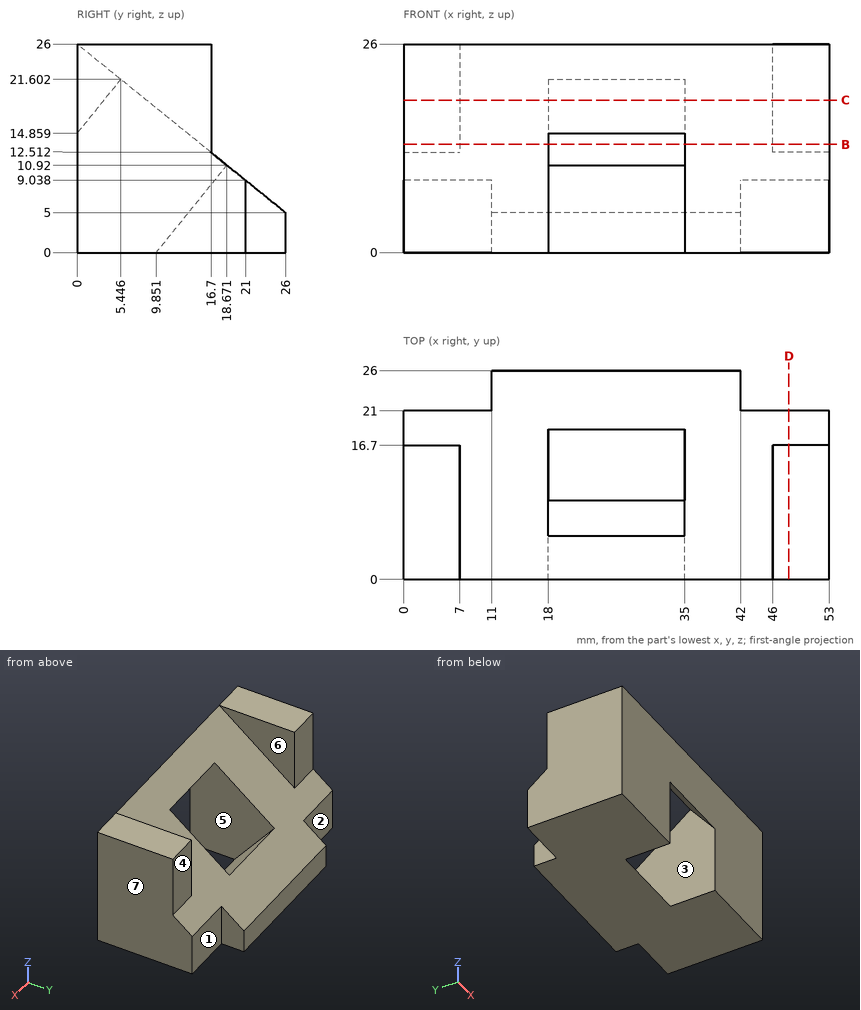
Could you check a few things on this drawing? It's one solid part, dimensions in mm from its lowest x, y, z. A direction names the side the tool comes from. Coordinates: 2 decimals unless noted, no trailing zeros. Order: outer loops, then holes, each group sorted by start corner. A loop starts at its lowest first (then second) coordinate and runs counter-clockwise, first axis right, second up.
1. For the marked faces 1, 2 and 3, which set-ups out of +Z, -Z, +X, -X, +Y, -Y let a thin tool reach every point of the face, with its end or its side?
2. If we section it at D-D (x = 48): Please give me the cut outline in (y, z).
3. If we section it at B-B (z = 13.5): Please give me the cut outline in (x, y), then the cut area to 3 significant figures.
4. I need wall thicknesses on line 1 (X direction, y = 12.25, z = 13.25); line 2 (X direction, y = 16.25, z = 15.75); line 3 (Z direction, x = 35.5, y = 20) (1 decimal). Which ranges of each line are inside material? Lowest first, please.
5. If we section it at C-C (z = 19): Please give me the cut outline in (x, y) (1 decimal).
6. I'm going to push flat-ended pins straight in: pin 1 (5.5 mm diameter, centred on x = 5, z = 17.5, fed in from +Y); pin 2 (1 mm diameter, centred on x = 11.5, z = 6, fed in from +Y); pin 3 (2.5 mm diameter, centred on x = 48.5, z = 5, fed in from +Y). Where does each tip first touch, or does it pass through?
7. Thinking about a two-plate mould opening in X: for the marked faces 4, 5, 6 and 7, which applies, +X half, -X half, draft (parallel to the pull), parting line (faces both ways), or undercut?
Entries:
1. face 1: +Z, -Z, +X, +Y
1. face 2: +Z, -Z, -X, +Y
1. face 3: none
2. outline: (0, 0) - (21, 0) - (21, 9.04) - (16.7, 12.51) - (16.7, 26) - (0, 26) - close
3. outline: (0, 0) - (18, 0) - (18, 15.48) - (7, 15.48) - (7, 16.7) - (0, 16.7) - close; (35, 0) - (53, 0) - (53, 16.7) - (46, 16.7) - (46, 15.48) - (35, 15.48) - close
3. area: 574 mm2
4. line 1: x = 0 to 18, 35 to 53
4. line 2: x = 0 to 7, 46 to 53
4. line 3: z = 0 to 9.8
5. outline: (0, 0) - (53, 0) - (53, 16.7) - (46, 16.7) - (46, 8.7) - (35, 8.7) - (35, 3.3) - (18, 3.3) - (18, 8.7) - (7, 8.7) - (7, 16.7) - (0, 16.7) - close
6. pin 1: stops at y = 16.7
6. pin 2: stops at y = 25.38
6. pin 3: stops at y = 21
7. face 4: draft
7. face 5: undercut
7. face 6: undercut
7. face 7: +X half
